The model under review builds one solid part; all positions refer to its coordinate system, in mm. A direction names the side the tool comes from. Round coordinates to 2 decimals unless told otherwise and drop trailing zeros. Order: outer loops, then holes, each group sorted by start corner. A loop starts at its lowest first (then second) coordinate and runs counter-clockwise, first axis right, second up. Notation, with made-up numbers: (46.25, 0) -> (80.25, 0) arc R17 cw to (80.25, 33) -> close; hole circle Ø11 at (77, 30). An arc over 180 degrees is marked (long way). Put each result on its own line as item: value. Start each with the question number.
from build123d import *

# Parameters (mm, degrees)
SKETCH1_W           = 52
SKETCH1_H           = 50
BOSS_EXTRUDE1_DEPTH = 13
SKETCH2_W           = 48
SKETCH2_H           = 46
CUT_EXTRUDE1_DEPTH  = 11
SKETCH3_W           = 6.1
SKETCH3_H           = 2
SKETCH3_W_2         = 8
CUT_EXTRUDE2_DEPTH  = 7
SKETCH4_W           = 3
SKETCH4_H           = 3
BOSS_EXTRUDE2_DEPTH = 3
SKETCH5_R           = 1
BOSS_EXTRUDE3_DEPTH = 11
SKETCH13_W          = 15
SKETCH13_H          = 2
CUT_EXTRUDE4_DEPTH  = 6
SKETCH12_R          = 20.065170359
CUT_EXTRUDE3_DEPTH  = 10


with BuildPart() as part:
    # Sketch1 → Boss-Extrude1 (new body)
    with BuildSketch(Plane(origin=(0, 0, 0), x_dir=(1, 0, 0), z_dir=(0, 1, 0))):
        with Locations((26, 25)):
            Rectangle(SKETCH1_W, SKETCH1_H)
    extrude(amount=BOSS_EXTRUDE1_DEPTH)

    # Sketch2 → Cut-Extrude1 (cut)
    with BuildSketch(Plane(origin=(0, 13, 0), x_dir=(1, 0, 0), z_dir=(0, 1, 0))):
        with Locations((26, 25)):
            Rectangle(SKETCH2_W, SKETCH2_H)
    extrude(amount=-CUT_EXTRUDE1_DEPTH, mode=Mode.SUBTRACT)

    # Sketch3 → Cut-Extrude2 (cut)
    with BuildSketch(Plane(origin=(0, 13, 0), x_dir=(1, 0, 0), z_dir=(0, 1, 0))):
        with Locations((40.05, 1)):
            Rectangle(SKETCH3_W, SKETCH3_H)
        with Locations((24.95, 1)):
            Rectangle(SKETCH3_W, SKETCH3_H)
        with Locations((12.8, 1)):
            Rectangle(SKETCH3_W_2, SKETCH3_H)
    extrude(amount=-CUT_EXTRUDE2_DEPTH, mode=Mode.SUBTRACT)

    # Sketch4 → Boss-Extrude2 (add)
    with BuildSketch(Plane(origin=(0, 2, 0), x_dir=(1, 0, 0), z_dir=(0, 1, 0))):
        with Locations((3.5, 46.5)):
            Rectangle(SKETCH4_W, SKETCH4_H)
        with Locations((48.5, 46.5)):
            Rectangle(SKETCH4_W, SKETCH4_H)
        with Locations((3.5, 3.5)):
            Rectangle(SKETCH4_W, SKETCH4_H)
        with Locations((48.5, 3.5)):
            Rectangle(SKETCH4_W, SKETCH4_H)
    extrude(amount=BOSS_EXTRUDE2_DEPTH)

    # Sketch5 → Boss-Extrude3 (add)
    with BuildSketch(Plane(origin=(0, 2, 0), x_dir=(1, 0, 0), z_dir=(0, 1, 0))):
        with Locations((50, 35)):
            Circle(SKETCH5_R)
        with Locations((50, 25)):
            Circle(SKETCH5_R)
        with Locations((50, 15)):
            Circle(SKETCH5_R)
        with Locations((50, 47)):
            Circle(SKETCH5_R)
        with Locations((50, 3)):
            Circle(SKETCH5_R)
    extrude(amount=BOSS_EXTRUDE3_DEPTH)

    # Sketch13 → Cut-Extrude4 (cut)
    with BuildSketch(Plane(origin=(0, 13, 0), x_dir=(1, 0, 0), z_dir=(0, 1, 0))):
        with Locations((38.5, 49)):
            Rectangle(SKETCH13_W, SKETCH13_H)
        with Locations((20, 49)):
            Rectangle(SKETCH13_W, SKETCH13_H)
    extrude(amount=-CUT_EXTRUDE4_DEPTH, mode=Mode.SUBTRACT)

    # Sketch12 → Cut-Extrude3 (cut)
    with BuildSketch(Plane(origin=(0, 2, 0), x_dir=(1, 0, 0), z_dir=(0, 1, 0))):
        with Locations(Location((26.189038813, 24.497096503, 0), (0, 0, 270))):
            Circle(SKETCH12_R)
    extrude(amount=-CUT_EXTRUDE3_DEPTH, mode=Mode.SUBTRACT)


solid = part.part
Q1. Take a section at D-D on y = 11. State how many separate pieces and enclosed holes the cut face has, and give its area (3 significant figures).
Q2. Take a section at A-A on z = -3. Give the boundary of the cut face in (x, y).
Q3. Clearance check with flat-ended pins moving along their axes: pin 1 Ø2 at (x, z) = (11.5, -1.5) entering from +Y; pin 2 Ø3 at (x, y) = (44, 9.5) entering from -Z. State where each tip first meets the part, or that it passes through.
Q4. For faces 1 (the face through (48, 5, -47)), 2 (the face through (38, 7, -49)), 3 (the face through (14, 0, -42)), list the 3-axis set-ups (+Z, -Z, +X, -X, +Y, -Y) from which the entire face can be reached by the end or side of a thin tool; tool diameter is ignored.
Q5. Take a section at C-C on z = -33. Give the boundary of the cut face in (x, y).
Q6. Take a section at B-B on x = 20.5. Give the boundary of the cut face in (y, z), and give its area (3 significant figures).
Q7. Draft analysis for pull direction Z (two halves, no side actions). For faces 4 (the face through (50, 8, -41)), 5 (the face through (25, 6, -1)), 6 (the face through (50, 8, -9)), state which applies: +Z half, -Z half, draft (parallel to the pull), parting line (faces both ways), or undercut.
Q8. Wall thickness on probe 1 along X at (y, z) = (9.25, -42); probe 2 along Z at (x, y) = (46.5, 2.75); probe 3 along X at (y, z) = (1.5, -25): over which ranges is each line inside the solid? List them lowest first. Write a range as [from, to].
Calculated:
1. separate pieces: 5
1. enclosed holes: 0
1. area: 299 mm²
2. outline: (0, 0) -> (52, 0) -> (52, 13) -> (49, 13) -> (49, 5) -> (47, 5) -> (47, 2) -> (5, 2) -> (5, 5) -> (2, 5) -> (2, 13) -> (0, 13) -> close
3. pin 1: stops at y = 6
3. pin 2: stops at z = -2
4. face 1: +Y
4. face 2: -Z, +Y
4. face 3: +Z, -Z, +X, -X, -Y
5. outline: (0, 0) -> (8.01, 0) -> (8.01, 2) -> (2, 2) -> (2, 13) -> (0, 13) -> close; (44.36, 0) -> (52, 0) -> (52, 13) -> (50, 13) -> (50, 2) -> (44.36, 2) -> close
6. outline: (0, -50) -> (7, -50) -> (7, -48) -> (2, -48) -> (2, -43.74) -> (0, -43.74) -> close; (0, -5.26) -> (2, -5.26) -> (2, -2) -> (13, -2) -> (13, 0) -> (0, 0) -> close
6. area: 55.0 mm²
7. face 4: undercut
7. face 5: draft
7. face 6: undercut
8. probe 1: x = [0, 2], [50, 52]
8. probe 2: z = [-50, -48], [-2, 0]
8. probe 3: x = [0, 6.13], [46.25, 52]
